Here's the drawing with two shaded views (mm, measured from the low corner). I have some questions. Coordinates: 2 decimals unless noted, no trailing zeros. Write each loop counter-clockwise with the first axis right and the second up, starting at its lowest first coordinate (ties: lowest second). Pieces come first, ordered by that corner, then holes.
Item 1: I want a section at D-D on y = 3. Please give me the cut outline in (x, z) (1 decimal), then the cut area to 3 significant figures.
Item 2: Thinking about a two-plate mould opening in Y: for the marked faces 1, 2 and 3, which applies, +Y half, -Y half, draft (parallel to the pull), parting line (faces both ways), or undercut?
Item 3: If I drill on probe 1 along Y at (x, z) = (22.5, 20); probe 2 along Y at (x, z) = (20, 16); probe 3 along X at (y, z) = (37, 35.5) (1 decimal), over which ranges is the centre line in solid material (lowest first)?
Item 4: I want a section at B-B on x = 15.5. Please give me the cut outline in (y, z).
Item 5: I want a section at A-A on y = 27. Please give me the cut outline in (x, z) (1 decimal).
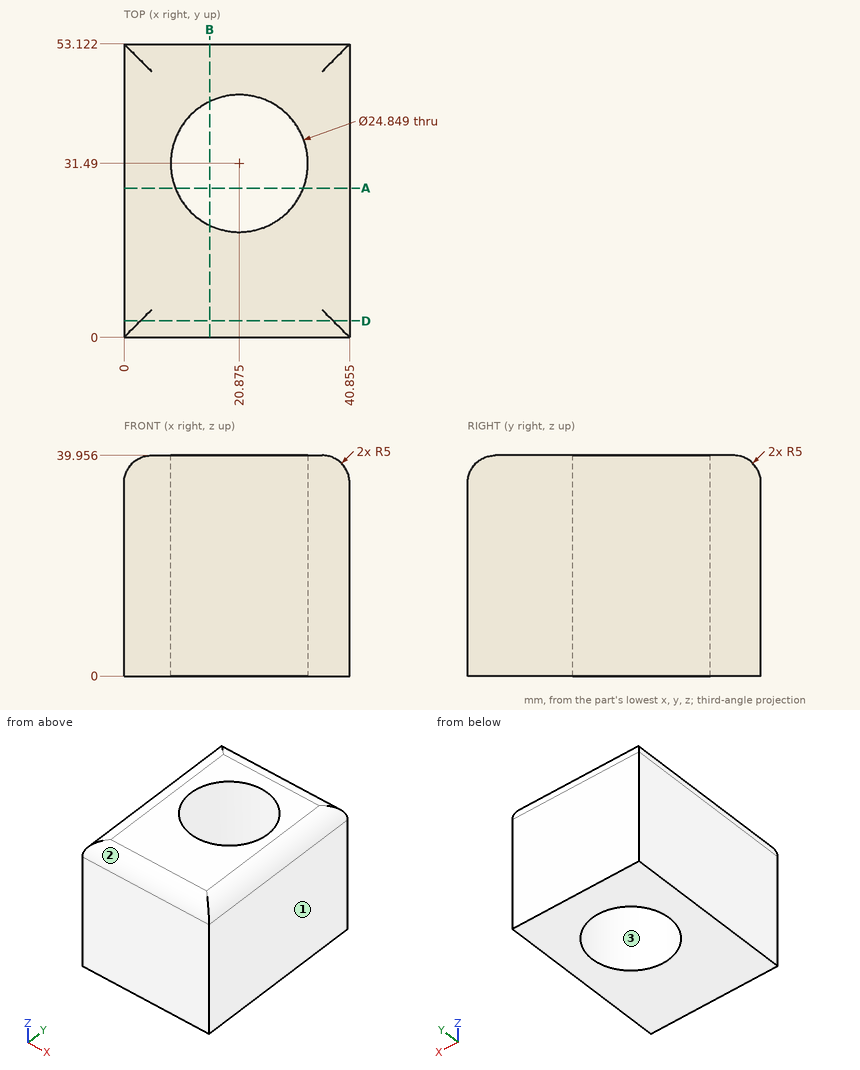
Response values:
1. outline: (0, 0) - (40.9, 0) - (40.9, 35) arc R5 ccw to (37.9, 39.5) - (3, 39.5) arc R5 ccw to (0, 35) - close
1. area: 1,610 mm2
2. face 1: draft
2. face 2: -Y half
2. face 3: undercut
3. probe 1: y = 0 to 19.17, 43.81 to 53.12
3. probe 2: y = 0 to 19.1, 43.88 to 53.12
3. probe 3: x = 0 to 9.7, 32 to 40.8
4. outline: (0, 0) - (20.29, 0) - (20.29, 39.96) - (5, 39.96) arc R5 ccw to (0, 34.96) - close; (42.69, 0) - (53.12, 0) - (53.12, 34.96) arc R5 ccw to (48.12, 39.96) - (42.69, 39.96) - close
5. outline: (0, 0) - (9.3, 0) - (9.3, 40) - (5, 40) arc R5 ccw to (0, 35) - close; (32.5, 0) - (40.9, 0) - (40.9, 35) arc R5 ccw to (35.9, 40) - (32.5, 40) - close
